CAD build for the part. Positions are in the model's coordinates, mm. A direction names the side the tool comes from. Coordinates: 2 decimals unless noted, no trailing zeros. Order: outer loops, then holes, each group sorted by start corner. A loop starts at its lowest first (then second) coordinate and runs counter-clockwise, first axis right, second up. Notation, with made-up numbers: M 41.5,86.25 L 57.5,86.25 A36 cw 57.5,120.25 Z; hole C 68,37.5 d1. An arc over 180 degrees is marked long. Write item = value, one per line.
from build123d import *

# Parameters (mm, degrees)
SKETCH1_R           = 2.1
BOSS_EXTRUDE1_DEPTH = 100


with BuildPart() as part:
    # Sketch1 → Boss-Extrude1 (new body)
    with BuildSketch(Plane(origin=(0, 0, 0), x_dir=(-1, 0, 0), z_dir=(0, 0, -1))):
        with BuildLine():
            Line((6, -8), (3, -8))
            Line((3, -8), (3, -10))
            Line((3, -10), (9, -10))
            ThreePointArc((9, -10), (9.707106781, -9.707106781), (10, -9))
            Line((10, -9), (10, -3))
            Line((10, -3), (8, -3))
            Line((8, -3), (8, -6))
            Line((8, -6), (7, -6))
            Line((7, -6), (4, -3))
            Line((4, -3), (4, 3))
            Line((4, 3), (7, 6))
            Line((7, 6), (8, 6))
            Line((8, 6), (8, 3))
            Line((8, 3), (10, 3))
            Line((10, 3), (10, 9))
            ThreePointArc((10, 9), (9.707106781, 9.707106781), (9, 10))
            Line((9, 10), (3, 10))
            Line((3, 10), (3, 8))
            Line((3, 8), (6, 8))
            Line((6, 8), (6, 7))
            Line((6, 7), (3, 4))
            Line((3, 4), (-3, 4))
            Line((-3, 4), (-6, 7))
            Line((-6, 7), (-6, 8))
            Line((-6, 8), (-3, 8))
            Line((-3, 8), (-3, 10))
            Line((-3, 10), (-9, 10))
            ThreePointArc((-9, 10), (-9.707106781, 9.707106781), (-10, 9))
            Line((-10, 9), (-10, 3))
            Line((-10, 3), (-8, 3))
            Line((-8, 3), (-8, 6))
            Line((-8, 6), (-7, 6))
            Line((-7, 6), (-4, 3))
            Line((-4, 3), (-4, -3))
            Line((-4, -3), (-7, -6))
            Line((-7, -6), (-8, -6))
            Line((-8, -6), (-8, -3))
            Line((-8, -3), (-10, -3))
            Line((-10, -3), (-10, -9))
            ThreePointArc((-10, -9), (-9.707106781, -9.707106781), (-9, -10))
            Line((-9, -10), (-3, -10))
            Line((-3, -10), (-3, -8))
            Line((-3, -8), (-6, -8))
            Line((-6, -8), (-6, -7))
            Line((-6, -7), (-3, -4))
            Line((-3, -4), (3, -4))
            Line((3, -4), (6, -7))
            Line((6, -7), (6, -8))
        make_face()
        with Locations(Location((0, 0, 0), (0, 0, 180))):
            Circle(SKETCH1_R, mode=Mode.SUBTRACT)
    extrude(amount=-BOSS_EXTRUDE1_DEPTH)


solid = part.part
(1) Pin check, flat tips, straight feed: pin 1 Ø5 at (x, z) = (1, 31.5) entering from -Y; pin 2 Ø0.6 at (x, z) = (-9.5, 32) entering from +Y. Stop position of each tip, or through.
Evaluation:
pin_1 = -10
pin_2 = 9.98
(2) Slice it at A-A, the plane y = 0. Write the cut outline in (x, z).
Evaluation:
outline = M -4,0 L -2.1,0 L -2.1,100 L -4,100 Z; M 2.1,0 L 4,0 L 4,100 L 2.1,100 Z
(3) Wall check: line 1 (Y direction, x = 0, z = 41.5); line 2 (Y direction, x = -9, z = 61.5); line 3 (Y direction, x = -4.25, z = 29.5). Give the ranges that are in metal, low to high. Write a range as from..to.
Evaluation:
line_1 = -4..-2.1, 2.1..4
line_2 = -10..-3, 3..10
line_3 = -10..-8, -5.25..-3.25, 3.25..5.25, 8..10
(4) Pull direction X, two halves, no side cores. Call faces 6 (the face through (10, 6, 49)), 7 (the face through (-3, 9, 49)), 8 (the face through (-10, 6, 49)): +X half, -X half, draft (parallel to the pull), parting line (faces both ways), or undercut.
Evaluation:
face_6 = +X half
face_7 = undercut
face_8 = -X half
(5) Tool access for faces 1 (the face through (9, 3, 49)), 2 (the face through (-9, 3, 49)), 3 (the face through (3, 9, 49)), 4 (the face through (-3, -9, 49)), 5 (the face through (-5, -8, 49)): list every direction of +Z, -Z, +X, -X, +Y, -Y with a clear straight run to the whole face (end or side of a thin tool).
Evaluation:
face_1 = +Z, -Z, +X
face_2 = +Z, -Z, -X
face_3 = +Z, -Z, +Y
face_4 = +Z, -Z, -Y
face_5 = +Z, -Z
